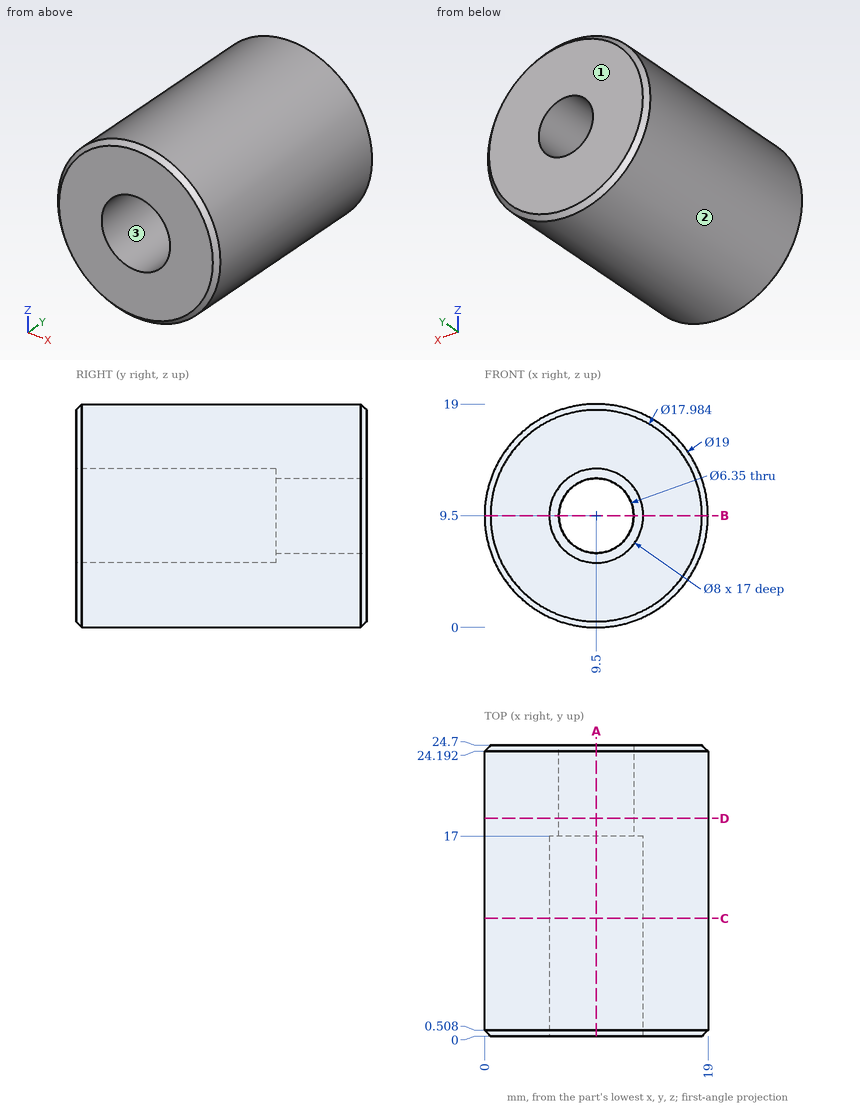
Answer from the drawing. Dimensions are ordinates in mm from the lowest x, y and z of the part. Round coordinates to 2 decimals unless told otherwise and drop trailing zeros. Loops run counter-clockwise (first coordinate to the right, second up) from the corner with the lowest first, then second, coordinate; pieces in that order, holes last.
(1) Find the intervals of material crossed by L1, parallel to Z at x = 9.5, y = 19.25 (3 decimals); L2, parallel to Z at x = 9.5, y = 13.5; L3, parallel to X at y = 22.5, z = 9.25, in increasing order.
Computed values:
L1: z = 0 to 6.325, 12.675 to 19
L2: z = 0 to 5.5, 13.5 to 19
L3: x = 0 to 6.33, 12.67 to 19
(2) The part is cut by section D-D, the plane y = 18.5. Give the vertices of the cut face in (x, z) (3 decimals).
Computed values:
outline: circle Ø19 at (9.5, 9.5); hole circle Ø6.35 at (9.5, 9.5)
(3) The part is cut by section B-B, the plane z = 9.5. Give the vertices of the cut face in (x, y) (3 decimals).
Computed values:
outline: (0, 0.508) - (0.508, 0) - (5.5, 0) - (5.5, 17) - (6.325, 17) - (6.325, 24.7) - (0.508, 24.7) - (0, 24.192) - close; (12.675, 17) - (13.5, 17) - (13.5, 0) - (18.492, 0) - (19, 0.508) - (19, 24.192) - (18.492, 24.7) - (12.675, 24.7) - close
(4) The part is cut by section A-A, the plane x = 9.5. Give the vertices of the cut face in (y, z) (3 decimals), and give its area (3 significant figures).
Computed values:
outline: (0, 0.508) - (0.508, 0) - (24.192, 0) - (24.7, 0.508) - (24.7, 6.325) - (17, 6.325) - (17, 5.5) - (0, 5.5) - close; (0, 13.5) - (17, 13.5) - (17, 12.675) - (24.7, 12.675) - (24.7, 18.492) - (24.192, 19) - (0.508, 19) - (0, 18.492) - close
area: 284 mm2
(5) The mould has two halves that part along X. Classify the marked faces 1, 2 and 3: pulls with the +X half, pulls with the -X half, needs draft (parallel to the pull), parting line crosses it, or undercut.
Computed values:
face 1: needs draft
face 2: parting line crosses it
face 3: undercut
(6) Each of these flat-tipped pins is pushed along its axis until it touches: P1, Ø1.5, axis at y = 9.5, z = 14, coming from the -X side; P2, Ø3, axis at y = 19.5, z = 10.5, coming from the -X side; P3, Ø4, axis at x = 3.5, y = 2.5, coming from the -Z side; P4, Ø3, axis at x = 16.5, y = 15.5, coming from the +Z side. Where does it stop, or does it pass through?
Computed values:
P1: stops at x = 0.77
P2: stops at x = 0
P3: stops at z = 0.88
P4: stops at z = 17.25
(7) The part is cut by section C-C, the plane y = 10. Give the vertices of the cut face in (x, z).
Computed values:
outline: circle Ø19 at (9.5, 9.5); hole circle Ø8 at (9.5, 9.5)
